Autodesk Inventor part; units mm, degrees
ref_plane "YZ Plane" through (0, 0, 0) normal (1, 0, 0) x (0, 1, 0)
ref_plane "XZ Plane" through (0, 0, 0) normal (0, 1, 0) x (-1, 0, 0)
ref_plane "XY Plane" through (0, 0, 0) normal (0, 0, 1) x (1, 0, 0)
sketch "Sketch1" plane through (0, 0, 0) normal (0, 1, 0) x (-1, 0, 0)
  line L0 (0, 0) -> (24, 0)
  line L1 (24, 0) -> (24, -53)
  line L2 (24, -53) -> (0, -53)
  line L3 (0, -53) -> (0, 0)
  dimension "d0" = 24
  dimension "d1" = 53
extrude "Extrusion1" add sketch "Sketch1" along normal blind 1
sketch "Sketch2" plane through (0, 1, 0) normal (0, 1, 0) x (1, 0, 0)
  line L0 (-24, 0) -> (0, 0)
  line L1 (0, 0) -> (0, 53)
  line L2 (-24, 53) -> (-24, 0)
  line L3 (-24, 0) -> (0, 0)
  line L4 (0, 0) -> (0, 1)
  line L5 (0, 1) -> (-24, 1)
  line L6 (-24, 1) -> (-24, 0)
  line L7 (0, 53) -> (-24, 53)
  line L8 (-24, 53) -> (-24, 52)
  line L9 (-24, 52) -> (0, 52)
  line L10 (0, 52) -> (0, 53)
  dimension "d4" = 1
  dimension "d5" = 1
extrude "Extrusion2" add sketch "Sketch2" along normal blind 40 contours L2 L5 L1 L0 | L2 L7 L1 L9
fillet "Fillet1" radius 12 4 edges at (0, 41, -52.5) (-24, 41, -52.5) (0, 41, -0.5) (-24, 41, -0.5)
sketch "Sketch3" plane through (0, 1, 0) normal (0, 1, 0) x (1, 0, 0)
  line L0 (0, 1) -> (0, 52)
  line L1 (-24, 52) -> (-24, 1)
  line L2 (-24, 26.5) -> (0, 26.5)
  circle A0 centre (-12, 26.5) radius 2.5
  point P0 (0, 0)
  dimension "d9" = 5
extrude "Extrusion3" cut sketch "Sketch3" against normal blind 40
properties part number "Wrist U-Plate"
Model file for the job. Use its own axes, mm. A direction names the side the tool comes from. Coordinates: 2 decimals unless noted, no trailing zeros. Order: outer loops, then holes, each group sorted by start corner. A loop starts at its lowest first (then second) coordinate and runs counter-clockwise, first axis right, second up. Notation, with made-up numbers: M 72,23 L 129,23 A17 ccw 129,55 Z; hole C 13.25,-30 d6. An arc over 180 degrees is marked long. Return JSON: item names as keys, results as strings.
1. Tool access for faces 5 (the face through (-3.61, 37.58, -0.51)), 6 (the face through (-12, 21, -1)): list every direction of +Z, -Z, +X, -X, +Y, -Y with a clear straight run to the whole face (end or side of a thin tool).
Ans:
{"face 5": "+Z, -Z, +X, +Y", "face 6": "+X, -X, +Y"}
2. Saw through at B-B (y = 11.5). Give the cut face in (x, z).
Ans:
{"outline": "M -24,-53 L 0,-53 L 0,-52 L -24,-52 Z; M -24,-1 L 0,-1 L 0,0 L -24,0 Z"}
3. Drill centre lines: probe 1 along Z at (x, y) = (-7, 16); probe 2 along Z at (x, y) = (-12, 0.8); probe 3 along X at (y, z) = (0.55, -26.5). Where is each one in solid material? Low to high.
Ans:
{"probe 1": "-53 to -52, -1 to 0", "probe 2": "-53 to -29, -24 to 0", "probe 3": "-24 to -14.5, -9.5 to 0"}
4. Saw through at C-C (x = -10.5). Give the cut face in (y, z), and give its area (3 significant figures).
Ans:
{"outline": "M 0,-53 L 40.91,-53 L 40.91,-52 L 1,-52 L 1,-28.5 L 0,-28.5 Z; M 0,-24.5 L 1,-24.5 L 1,-1 L 40.91,-1 L 40.91,0 L 0,0 Z", "area": "129 mm^2"}
5. Saw through at A-A (z = -26.5). Give the cut face in (x, y), and give its area (3 significant figures).
Ans:
{"outline": "M -24,0 L -14.5,0 L -14.5,1 L -24,1 Z; M -9.5,0 L 0,0 L 0,1 L -9.5,1 Z", "area": "19.0 mm^2"}
6. Pull direction Z, two halves, no side cores. Call faces 1 (the face through (-12.33, 0.51, -28.98)), 2 (the face through (-9, 0, -26)), 3 (the face through (-12, 20, -53)), 4 (the face through (-12, 20, 0)): +Z half, -Z half, draft (parallel to the pull), parting line (faces both ways), or undercut.
Ans:
{"face 1": "undercut", "face 2": "draft", "face 3": "-Z half", "face 4": "+Z half"}
7. Saw through at D-D (x = -2). Give the cut face in (y, z).
Ans:
{"outline": "M 0,-53 L 35.63,-53 L 35.63,-52 L 1,-52 L 1,-1 L 35.63,-1 L 35.63,0 L 0,0 Z"}
8. Flat gauge pin, fed straight in: pin 1 (1.5 mm diameter, centred on x = -20.5, z = -6.5, fed in from +Y). Where does the tip first touch, or does it go through?
Ans:
{"pin 1": "y = 1"}
